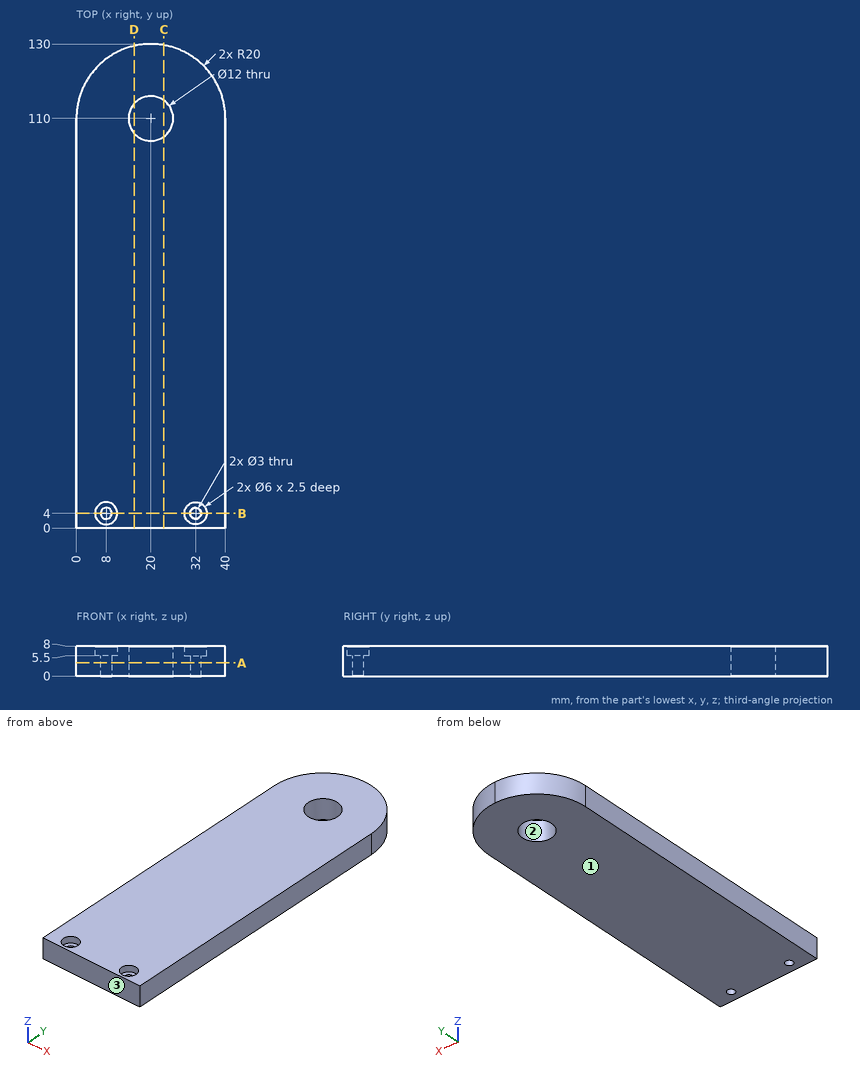
Here's the drawing with two shaded views (mm, measured from the low corner). I have some questions. Give positions to 0.01 mm unless a question says otherwise; leave off trailing zeros. Loops run counter-clockwise (first coordinate to the right, second up) from the corner with the lowest first, then second, coordinate; pieces in that order, holes last. Notation, with made-up numbers: M 80,67 L 97,67 A28 ccw 97,104 Z; hole C -24.75,84.25 d11. An arc over 180 degrees is marked long. One line per item, written item: value. Start each with the question number.
1) If we section it at C-C, the plane x = 23.5: Write out the boundary of the cut face in (y, z).
2) I'm going to push a flat-ended pin straight in: pin 1 (3 mm diameter, centred on x = 8.5, y = 4.5, fed in from +Z). Where does the tip first touch, or does it pass through?
3) Thinking about a two-plate mould opening in Y: for the marked faces 1, 2 and 3, which applies, +Y half, -Y half, draft (parallel to the pull), parting line (faces both ways), or undercut?
4) If we section it at B-B, the plane y = 4: Write out the boundary of the cut face in (x, z), and give its area (3 significant figures).
5) If we section it at A-A, the plane z = 3.5: Give the number of separate pieces and of enclosed holes in the cut face, and give its area (3 significant figures).
6) If I drill on line 1 (Y direction, x = 8, z = 6); line 2 (Y direction, x = 7.5, z = 7.25) (1 decimal); line 3 (X direction, y = 119, z = 3.5), over which ranges is the centre line in solid material (lowest first)? Write a range as [from, to].
7) If we section it at D-D, the plane x = 15.5: Write out the boundary of the cut face in (y, z).
Completed:
1. outline: M 0,0 L 105.13,0 L 105.13,8 L 0,8 Z; M 114.87,0 L 129.69,0 L 129.69,8 L 114.87,8 Z
2. pin 1: stops at z = 5.5
3. face 1: draft
3. face 2: undercut
3. face 3: -Y half
4. outline: M 0,0 L 6.5,0 L 6.5,5.5 L 5,5.5 L 5,8 L 0,8 Z; M 9.5,0 L 30.5,0 L 30.5,5.5 L 29,5.5 L 29,8 L 11,8 L 11,5.5 L 9.5,5.5 Z; M 33.5,0 L 40,0 L 40,8 L 35,8 L 35,5.5 L 33.5,5.5 Z
4. area: 257 mm^2
5. separate pieces: 1
5. enclosed holes: 3
5. area: 4,900 mm^2
6. line 1: y = [0, 1], [7, 126]
6. line 2: y = [0, 1], [7, 125.6]
6. line 3: x = [2.14, 37.86]
7. outline: M 0,0 L 106.03,0 L 106.03,8 L 0,8 Z; M 113.97,0 L 129.49,0 L 129.49,8 L 113.97,8 Z
